Model file for the job. Use its own axes, mm. A direction names the side the tool comes from. Round coordinates to 2 decimals unless told otherwise and drop trailing zeros. Loops run counter-clockwise (first coordinate to the right, second up) from the corner with the lowest first, then second, coordinate; pieces in that order, holes last. Notation, with made-up numbers: M 40.5,51 L 81.5,51 A26 cw 81.5,87 Z; hole C -26.75,53 d11. An arc over 180 degrees is marked long. Answer in a Markdown table with one row per item.
from build123d import *

# Parameters (mm, degrees)
CROQUIS1_R                 = 30
CROQUIS1_R_2               = 1.99901262
SALIENTE_EXTRUIR1_DEPTH    = 4
CROQUIS2_W                 = 40.0311451
CROQUIS2_H                 = 42.320959557
SALIENTE_EXTRUIR2_DEPTH    = 150
CORTAR_EXTRUIR1_REACH      = 52.016
CROQUIS3_R                 = 3.2
CROQUIS4_W                 = 33.4
CROQUIS4_H                 = 13
CORTAR_EXTRUIR2_DEPTH      = 12
CROQUIS5_W                 = 21.241045897
CROQUIS5_H                 = 13
CORTAR_EXTRUIR3_DEPTH      = 17
CROQUIS6_R                 = 1
CORTAR_EXTRUIR4_DEPTH      = 5
CORTAR_EXTRUIR6_DEPTH      = 10.98442745
CORTAR_EXTRUIR6_DEPTH_BACK = 51.01557255
CROQUIS10_R                = 3.2
CORTAR_EXTRUIR10_DEPTH     = 10
CROQUIS11_W                = 14
CROQUIS11_H                = 13
CORTAR_EXTRUIR11_DEPTH     = 6.1
CROQUIS12_W                = 10
CROQUIS12_H                = 9.978436174
CORTAR_EXTRUIR12_DEPTH     = 17
CROQUIS13_W                = 10
CROQUIS13_H                = 10
CORTAR_EXTRUIR13_DEPTH     = 45
CROQUIS11_3_W              = 14
CROQUIS11_3_H              = 13
CORTAR_EXTRUIR18_DEPTH     = 27.3


with BuildPart() as part:
    # Croquis1 → Saliente-Extruir1 (new body)
    with BuildSketch(Plane.XY):
        Circle(CROQUIS1_R)
        with Locations((27.5, 0)):
            Circle(CROQUIS1_R_2, mode=Mode.SUBTRACT)
        with Locations((0, -27.5)):
            Circle(CROQUIS1_R_2, mode=Mode.SUBTRACT)
        with Locations((-27.5, 0)):
            Circle(CROQUIS1_R_2, mode=Mode.SUBTRACT)
        with Locations((0, 27.5)):
            Circle(CROQUIS1_R_2, mode=Mode.SUBTRACT)
    extrude(amount=SALIENTE_EXTRUIR1_DEPTH)

    # Croquis2 → Saliente-Extruir2 (add)
    with BuildSketch(Plane.XY.offset(4)):
        with Locations((0, -1.186261717)):
            Rectangle(CROQUIS2_W, CROQUIS2_H)
    extrude(amount=SALIENTE_EXTRUIR2_DEPTH)

    # Croquis3 → Cortar-Extruir1 (cut, up to next)
    with BuildSketch(Plane.ZY.offset(20.01557255), mode=Mode.PRIVATE) as cortar_extruir1_sk1:
        with Locations((36, -11.961033968)):
            Circle(CROQUIS3_R)
    cortar_extruir1_tool1 = extrude(cortar_extruir1_sk1.sketch, amount=-CORTAR_EXTRUIR1_REACH, mode=Mode.PRIVATE) & part.part
    add(cortar_extruir1_tool1.solids().sort_by_distance((-20.015573, -11.961034, 36))[0], mode=Mode.SUBTRACT)

    # Croquis4 → Cortar-Extruir2 (cut)
    with BuildSketch(Plane.ZY.offset(20.01557255)):
        with Locations((76.773642677, -11.961033968)):
            Rectangle(CROQUIS4_W, CROQUIS4_H)
    extrude(amount=-CORTAR_EXTRUIR2_DEPTH, mode=Mode.SUBTRACT)

    # Croquis5 → Cortar-Extruir3 (cut)
    with BuildSketch(Plane.ZY.offset(8.01557255)):
        with Locations((76.753119728, -11.961033968)):
            Rectangle(CROQUIS5_W, CROQUIS5_H)
    extrude(amount=-CORTAR_EXTRUIR3_DEPTH, mode=Mode.SUBTRACT)

    # Croquis6 → Cortar-Extruir4 (cut)
    with BuildSketch(Plane.ZY.offset(8.01557255)):
        with Locations((63.103119729, -11.961033968)):
            Circle(CROQUIS6_R)
        with Locations((90.423642677, -11.961033968)):
            Circle(CROQUIS6_R)
    extrude(amount=-CORTAR_EXTRUIR4_DEPTH, mode=Mode.SUBTRACT)

    # Croquis7 → Cortar-Extruir6 (cut, two sides)
    with BuildSketch(Plane.ZY.offset(20.01557255)) as cortar_extruir6_sk:
        Polygon((102.262078688, -22.346741496), (154, -22.346741496), (154, 19.974218061), (79, 19.974218061), (102.262078688, 11.767260679), align=None)
    extrude(amount=CORTAR_EXTRUIR6_DEPTH, mode=Mode.SUBTRACT)
    extrude(cortar_extruir6_sk.sketch, amount=-CORTAR_EXTRUIR6_DEPTH_BACK, mode=Mode.SUBTRACT)

    # Croquis10 → Cortar-Extruir10 (cut)
    with BuildSketch(Plane(origin=(20.01557255, 0, 0), x_dir=(0, 0, -1), z_dir=(1, 0, 0))):
        with Locations((-72, -11.961033968)):
            Circle(CROQUIS10_R)
    extrude(amount=-CORTAR_EXTRUIR10_DEPTH, mode=Mode.SUBTRACT)

    # Croquis11 → Cortar-Extruir11 (cut)
    with BuildSketch(Plane.XY.offset(66.13259678)):
        with Locations((1.98442745, -11.961033968)):
            Rectangle(CROQUIS11_W, CROQUIS11_H)
    extrude(amount=-CORTAR_EXTRUIR11_DEPTH, mode=Mode.SUBTRACT)

    # Croquis12 → Cortar-Extruir12 (cut)
    with BuildSketch(Plane.XY.offset(60.03259678)):
        with Locations((3.98442745, -11.950252055)):
            Rectangle(CROQUIS12_W, CROQUIS12_H)
    extrude(amount=-CORTAR_EXTRUIR12_DEPTH, mode=Mode.SUBTRACT)

    # Croquis13 → Cortar-Extruir13 (cut)
    with BuildSketch(Plane.XZ.offset(6.961033968)):
        with Locations((3.98442745, 48.03259678)):
            Rectangle(CROQUIS13_W, CROQUIS13_H)
    extrude(amount=-CORTAR_EXTRUIR13_DEPTH, mode=Mode.SUBTRACT)

    # Croquis11_3 → Cortar-Extruir18 (cut)
    with BuildSketch(Plane.XY.offset(66.13259678)):
        with Locations((1.98442745, -11.961033968)):
            Rectangle(CROQUIS11_3_W, CROQUIS11_3_H)
    extrude(amount=CORTAR_EXTRUIR18_DEPTH, mode=Mode.SUBTRACT)


solid = part.part
1. Pin check, flat tips, straight feed: pin 1 (3 mm diameter, centred on y = -11.96, z = 90.42, fed in from +X); pin 2 (6 mm diameter, centred on y = -12.5, z = 11, fed in from -X); pin 3 (8 mm diameter, centred on x = -18, z = 12.5, fed in from +Y). Stop position of each tip, or through.
Verdict:
| item | result |
|---|---|
| pin 1 | stops at x = 20.02 |
| pin 2 | stops at x = -20.02 |
| pin 3 | stops at y = 19.97 |
2. Mould opens along Z. For faces 1 (the cylindrical face through (0.922, -29.273, 1.972)), 2 (the flat face through (2, -12, 93.433)), 3 (the flat face through (-5, 21, 4)) say: +Z half, -Z half, draft (parallel to the pull), parting line (faces both ways), or undercut.
Verdict:
| item | result |
|---|---|
| face 1 | draft |
| face 2 | undercut |
| face 3 | +Z half |
3. Saw through at C-C (x = 5.5). Write the cut outline in (y, z), and give its area (3 significant figures).
Verdict:
| item | result |
|---|---|
| outline | M -29.49,0 L 29.49,0 L 29.49,4 L 19.97,4 L 19.97,43.03 L -16.94,43.03 L -16.94,60.03 L -18.46,60.03 L -18.46,93.43 L -5.46,93.43 L -5.46,60.03 L -6.96,60.03 L -6.96,53.03 L 19.97,53.03 L 19.97,79 L 11.77,102.26 L -22.35,102.26 L -22.35,4 L -29.49,4 Z; hole C -11.96,36 d6.4 |
| area | 3,390 mm² |
4. Wall check: probe 1 along Z at (x, y) = (2, -5.5); probe 2 along Z at (x, y) = (-4, -12); probe 3 along Y at (x, z) = (-7, 36). Give the ranges that are in metal, low to high.
Verdict:
| item | result |
|---|---|
| probe 1 | z = 0 to 43.03, 53.03 to 60.03, 93.43 to 102.26 |
| probe 2 | z = 0 to 32.8, 39.2 to 60.03, 93.43 to 102.26 |
| probe 3 | y = -22.35 to -15.16, -8.76 to 19.97 |
5. Saw through at D-D (z = 77). Write the cut outline in (x, y), and give its area (3 significant figures).
Verdict:
| item | result |
|---|---|
| outline | M -20.02,-22.35 L 20.02,-22.35 L 20.02,19.97 L -20.02,19.97 L -20.02,-5.46 L 8.98,-5.46 L 8.98,-18.46 L -20.02,-18.46 Z |
| area | 1,320 mm² |
6. Tool access for faces 4 (the flat face through (-14, -12, 93.474)), 5 (the flat face through (0, -22.347, 52)), 6 (the flat face through (4, 6, 53.033)), 7 (the flat face through (-5.016, -12, 92)): list every direction of +Z, -Z, +X, -X, +Y, -Y with a clear straight run to the whole face (end or side of a thin tool).
Verdict:
| item | result |
|---|---|
| face 4 | -X |
| face 5 | +Z, +X, -X, -Y |
| face 6 | +Y |
| face 7 | none |
7. Saw through at B-B (x = -27.5). Write the cut outline in (y, z), and give its area (3 significant figures).
Verdict:
| item | result |
|---|---|
| outline | M -11.99,0 L -2,0 L -2,4 L -11.99,4 Z; M 2,0 L 11.99,0 L 11.99,4 L 2,4 Z |
| area | 79.9 mm² |
8. Saw through at A-A (z = 36). Write the cut outline in (x, y).
Verdict:
| item | result |
|---|---|
| outline | M -20.02,-22.35 L 20.02,-22.35 L 20.02,-15.16 L -20.02,-15.16 Z; M -20.02,-8.76 L 20.02,-8.76 L 20.02,19.97 L -20.02,19.97 Z |
